from build123d import *

# Parameters (mm, degrees)
F0_W     = 22.86
F0_H     = 18.415
F1_DEPTH = 1.651
F2_W     = 7.9502
F2_H     = 6.8834
F3_DEPTH = 3.175
F4_W     = 9.525
F4_H     = 7.62
F5_DEPTH = 4.064
F6_R     = 1.27
F7_DEPTH = 3.175


with BuildPart() as f1:
    # F0 (on Top) → F1 (new body)
    with BuildSketch(Plane.XY):
        Rectangle(F0_W, F0_H)
    extrude(amount=F1_DEPTH)

    # F2 (on face) → F3 (join)
    with BuildSketch(Plane.XY.offset(1.651)):
        with Locations((-7.4549, 5.7658)):
            Rectangle(F2_W, F2_H)
    extrude(amount=F3_DEPTH)

    # F4 (on Top) → F5 (join)
    with BuildSketch(Plane.XY):
        with Locations((-6.068009, -4.990071)):
            Rectangle(F4_W, F4_H)
    extrude(amount=-F5_DEPTH)

    # F6 (on face) → F7 (cut)
    with BuildSketch(Plane(origin=(0, 0, -4.064), x_dir=(1, 0, 0), z_dir=(0, 0, -1))):
        with Locations((-6.068009, 4.990071)):
            Circle(F6_R)
    extrude(amount=-F7_DEPTH, mode=Mode.SUBTRACT)


solid = f1.part
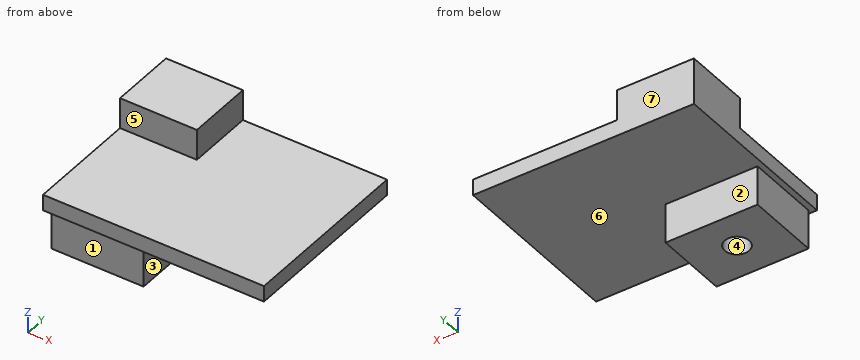
Could you check a few things on this model? Use its own coordinates, in mm. Face numbers are marked on the shaded views. A direction names the side the tool comes from. Round coordinates to 2 decimals unless told otherwise and drop trailing zeros. Order: outer loops, then holes, each group sorted by start corner. A loop starts at its lowest first (then second) coordinate and runs counter-clockwise, first axis right, second up.
Q1. Imagine slicing it at D-D, the plane z = -2. List the corners of the cut face in (x, y) for me, then the cut area to 3 significant figures.
Geometry says:
outline: (-10.83, -8.8) - (-1.31, -8.8) - (-1.31, -1.18) - (-10.83, -1.18) - close; hole circle Ø2.54 at (-6.07, -4.99)
area: 67.5 mm2
Q2. Imagine slicing it at A-A, the plane y = -2.5. List the corners of the cut face in (x, z) for me, then the cut area to 3 significant figures.
Geometry says:
outline: (-11.43, 0) - (-10.83, 0) - (-10.83, -4.06) - (-1.31, -4.06) - (-1.31, 0) - (11.43, 0) - (11.43, 1.65) - (-11.43, 1.65) - close
area: 76.5 mm2
Q3. I'm going to push flat-ended pins straight in: P1, Ø3.5, axis at x = -6.07, y = -4.99, coming from the +Z side; P2, Ø1.6, axis at x = -8.5, z = 4, coming from the -Y side; P3, Ø1.2, axis at y = -5.5, z = -3, coming from the -X side. Where does each tip first touch, or does it pass through?
Geometry says:
P1: stops at z = 1.65
P2: stops at y = 2.32
P3: stops at x = -10.83
Q4. Which directions (+Z, -Z, +X, -X, +Y, -Y) give clear straight access to the entire face, cutting with the end or side of a thin tool? Please do the marked faces 1, 2 and 3.
Geometry says:
face 1: -Z, +X, -X, -Y
face 2: -Z, +X, -X, +Y
face 3: -Z, +X, +Y, -Y
Q5. Imagine slicing it at C-C, the plane z = 2.25. List the corners of the cut face in (x, y) for me.
Geometry says:
outline: (-11.43, 2.32) - (-3.48, 2.32) - (-3.48, 9.21) - (-11.43, 9.21) - close
Q6. Thinking about a two-plate mould opening in Y: for the marked faces 4, 5, 6 and 7, which applies, released by +Y, released by -Y, zero draft, split by the parting line, or undercut?
Geometry says:
face 4: undercut
face 5: released by -Y
face 6: zero draft
face 7: released by +Y
Q7. Imagine slicing it at B-B, the plane x = -2. List the corners of the cut face in (y, z) for me.
Geometry says:
outline: (-9.21, 0) - (-8.8, 0) - (-8.8, -4.06) - (-1.18, -4.06) - (-1.18, 0) - (9.21, 0) - (9.21, 1.65) - (-9.21, 1.65) - close
Q8. Please list where these lines run through material, in increasing order: probe 1 along Z at (x, y) = (6.5, 0.5); probe 2 along X at (y, z) = (-4.5, -2.75); probe 3 along Z at (x, y) = (-6, 7).
Geometry says:
probe 1: z = 0 to 1.65
probe 2: x = -10.83 to -7.24, -4.9 to -1.31
probe 3: z = 0 to 4.83
